```python
from build123d import *

# Parameters (mm, degrees)
F0_W          = 355.6
F0_H          = 508
F1_DEPTH      = 381
F4_DEPTH      = 101.6
F4_DEPTH_BACK = 101.6
F5_DEPTH      = 127
F5_DEPTH_BACK = 127


with BuildPart() as f1:
    # F0 (on Top) → F1 (new body)
    with BuildSketch(Plane.XY):
        with Locations((177.8, 254)):
            Rectangle(F0_W, F0_H)
    extrude(amount=F1_DEPTH)

    # F3 (on mid) → F4 (join, two sides)
    with BuildSketch(Plane(origin=(177.8, 0, 0), x_dir=(0, -1, 0), z_dir=(-1, 0, 0))) as f4_sk:
        with BuildLine():
            ThreePointArc((77.2475148298, 158.7932740141), (63.5, 171.45), (77.2475148298, 184.1067259859))
            Line((77.2475148298, 184.1067259859), (0, 190.5))
            Line((0, 190.5), (0, 152.4))
            Line((0, 152.4), (77.2475148298, 158.7932740141))
        make_face()
    extrude(amount=F4_DEPTH)
    extrude(f4_sk.sketch, amount=-F4_DEPTH_BACK)

    # F3 (on mid) → F5 (join, two sides)
    with BuildSketch(Plane(origin=(177.8, 0, 0), x_dir=(0, -1, 0), z_dir=(-1, 0, 0))) as f5_sk:
        with BuildLine():
            ThreePointArc((77.2475148298, 158.7932740141), (85.5432713312, 162.8480652856), (88.9, 171.45))
            ThreePointArc((88.9, 171.45), (85.5432713312, 180.0519347144), (77.2475148298, 184.1067259859))
            ThreePointArc((77.2475148298, 184.1067259859), (63.5, 171.45), (77.2475148298, 158.7932740141))
        make_face()
    extrude(amount=F5_DEPTH)
    extrude(f5_sk.sketch, amount=-F5_DEPTH_BACK)


solid = f1.part
```
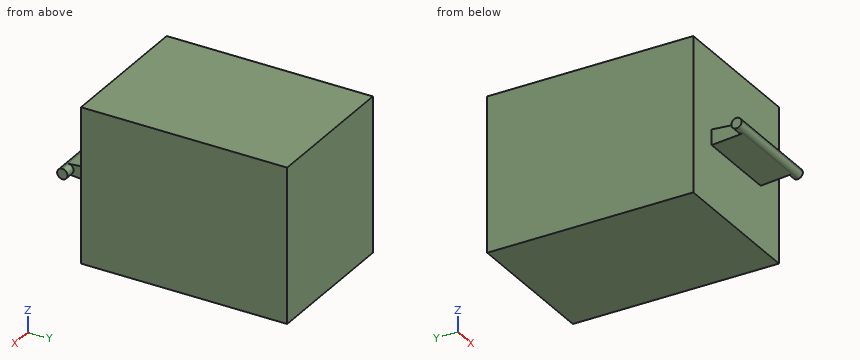
Geometry: final body of the model. Coordinates: model frame, mm. Round coordinates to 2 decimals unless told otherwise and drop trailing zeros. Write each loop counter-clockwise with the first axis right and the second up, starting at its lowest first coordinate (ties: lowest second). Pieces come first, ordered by that corner, then holes. Notation, with made-up numbers: M 27,-26.5 L 66,-26.5 A21 cw 66,-6.5 Z; hole C -40,82 d3. An arc over 180 degrees is marked long. Answer in a Markdown table with one row per item. Add a question column.
(1) Cut plane A-A, the plane x = 262. Return the cut outline in (y, z).
(2) Contact query for flat-ended pins moving along their axis: pin 1 (11.5 mm diameter, centred on y = -42, z = 167, fed in from -X); pin 2 (7.5 mm diameter, centred on y = -78, z = 175.5, fed in from -X); pin 3 (7.5 mm diameter, centred on y = -76.5, z = 170, fed in from +X). Output: stop coordinate, or through.
(3) Cut plane C-C, the plane z = 233.5. Return the cut outline in (x, y).
(4) Cut plane B-B, the plane x = 67.5. Return the cut outline in (y, z).
(5) Cut plane D-D, the plane y = -46. Return the cut outline in (x, z), then the cut area to 3 significant figures.
(6) Ray query, L1, parallel to Y at x = 315, z = 219; L2, parallel to Z at x = 166.5, y = -39.5; L3, parallel to Z at x = 260, y = -64. Return the intervals inside material, ascending.
Established:
| question | item | result |
|---|---|---|
| 1 | outline | M -77.25,158.79 L 0,152.4 L 0,0 L 508,0 L 508,381 L 0,381 L 0,190.5 L -77.25,184.11 A12.7 ccw Z |
| 2 | pin 1 | x = 76.2 |
| 2 | pin 2 | x = 50.8 |
| 2 | pin 3 | x = 304.8 |
| 3 | outline | M 0,0 L 355.6,0 L 355.6,508 L 0,508 Z |
| 4 | outline | C -76.2,171.45 d25.4; M 0,0 L 508,0 L 508,381 L 0,381 Z |
| 5 | outline | M 76.2,156.21 L 279.4,156.21 L 279.4,186.69 L 76.2,186.69 Z |
| 5 | area | 6,190 mm² |
| 6 | L1 | 0 to 508 |
| 6 | L2 | 155.67 to 187.23 |
| 6 | L3 | 157.7 to 185.2 |
